Verification items for this drawing (mm, ordinates from the low corner). A direction names the side the tool comes from. Coordinates: 2 decimals unless noted, no trailing zeros. Write each loop counter-clockwise with the first axis right and the second up, starting at its lowest first coordinate (ties: lowest second). Pieces come first, ordered by that corner, then holes. Notation, with made-up numbers: (51.5, 72) -> (100.5, 72) arc R36 ccw to (100.5, 107) -> close; hole circle Ø4 at (35, 19.5). An arc over 180 degrees is marked (long way). One line per item, written item: value. Start each with the question number.
1) Sectioned sample at B-B on y = 50. Give the number of separate pieces and of enclosed holes in the cut face, plus the area to 3 significant figures.
2) Draft check along X on the marked faces 1, 2 and 3. Enter one of: +X half, -X half, draft (parallel to the pull), parting line (faces both ways), or undercut.
3) Sectioned sample at C-C on z = 5. Enter the section's corners in (x, y).
4) Sectioned sample at D-D on y = 10. Enter the section's corners in (x, z), plus the area to 3 significant figures.
5) Sectioned sample at A-A on x = 50. Enter the section's corners in (y, z).
6) Gauge pin test, flat ends, axial feed: P1, Ø0.9, axis at y = 13, z = 1.5, coming from the -X side; P2, Ø2, axis at x = 27.5, z = 5, coming from the +Y side; P3, Ø8.5, axis at x = 50, y = 50, coming from the +Z side; P4, Ø5, axis at x = 30, y = 10, coming from the -Z side. Record the tip position at first contact, or that the pin passes through.
7) Set-up check for the marked faces 4, 5 and 6: record each of +Z, -Z, +X, -X, +Y, -Y from which the full face is reachable in a straight line by a thin tool's end or side.
8) Scan lines: line 1 along X through (y, z) = (48, 4.25); line 2 along Y through (x, z) = (33.5, 4); line 3 along Y through (x, z) = (30, 3.3). Record each from-to range of solid material in increasing order. Write a range as [from, to].
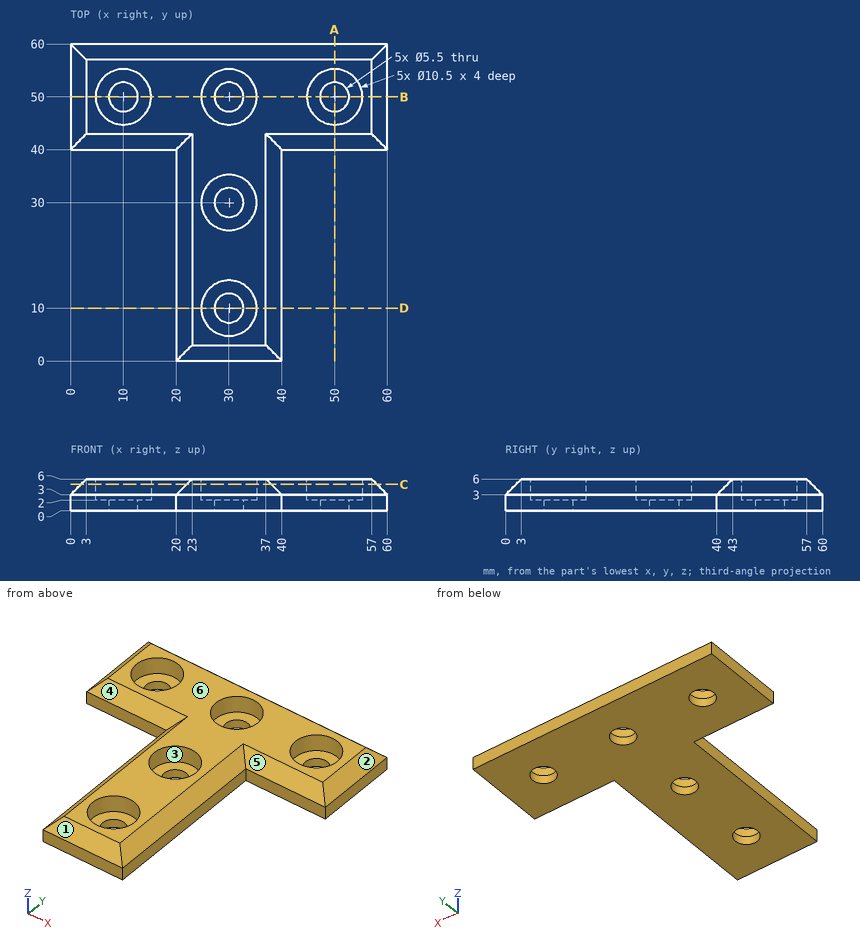
Answers:
1. separate pieces: 4
1. enclosed holes: 0
1. area: 192 mm2
2. face 1: draft
2. face 2: +X half
2. face 3: undercut
3. outline: (2, 42) -> (22, 42) -> (22, 2) -> (38, 2) -> (38, 42) -> (58, 42) -> (58, 58) -> (2, 58) -> close; hole circle Ø10.5 at (10, 50); hole circle Ø10.5 at (30, 10); hole circle Ø10.5 at (30, 30); hole circle Ø10.5 at (30, 50); hole circle Ø10.5 at (50, 50)
4. outline: (20, 0) -> (27.25, 0) -> (27.25, 2) -> (24.75, 2) -> (24.75, 6) -> (23, 6) -> (20, 3) -> close; (32.75, 0) -> (40, 0) -> (40, 3) -> (37, 6) -> (35.25, 6) -> (35.25, 2) -> (32.75, 2) -> close
4. area: 58.0 mm2
5. outline: (40, 0) -> (47.25, 0) -> (47.25, 2) -> (44.75, 2) -> (44.75, 6) -> (43, 6) -> (40, 3) -> close; (52.75, 0) -> (60, 0) -> (60, 3) -> (57, 6) -> (55.25, 6) -> (55.25, 2) -> (52.75, 2) -> close
6. P1: stops at x = 20
6. P2: stops at y = 59
6. P3: stops at z = 2
6. P4: passes through
7. face 4: +Z, -X, -Y
7. face 5: +Z, +X, -Y
7. face 6: +Z, +X, -X, +Y, -Y
8. line 1: x = [1.25, 5.15], [14.85, 25.15], [34.85, 45.15], [54.85, 58.75]
8. line 2: y = [1, 6.09], [13.91, 26.09], [33.91, 46.09], [53.91, 59]
8. line 3: y = [0.3, 4.75], [15.25, 24.75], [35.25, 44.75], [55.25, 59.7]
